For this review, take the finished solid that the model builds, in its own axes (mm). A direction names the side the tool comes from. Round coordinates to 2 decimals unless told otherwise and drop trailing zeros. Loops run counter-clockwise (first coordinate to the right, second up) from the corner with the lowest first, then second, coordinate; pieces in that order, holes last. Notation, with made-up numbers: (20, -39) -> (38, -39) arc R17 cw to (38, -29) -> close; hole circle Ø3 at (48, -9). An arc over 180 degrees is marked (long way). One line per question, with ' | ' between items. Start each with the question number.
1. Consider section C-C (x = -10.5). Write out the cut boundary in (y, z).
2. For pin 1 Ø8 at (x, y) = (11.5, 5) entering from -Z, flat-tipped, find the tip position at first contact; note if it passes through.
3. Wall thickness on line 1 along Y through (x, z) = (-2, 90.5); line 2 along X through (y, z) = (11.75, 30): over which ranges is each line inside the solid? List them lowest first.
4. For faces 1 (the face through (11.1, 11.14, 105.49)), 2 (the face through (-13.196, -13.289, 105.49)), list the 3-axis set-ups (+Z, -Z, +X, -X, +Y, -Y) from which the entire face can be reached by the end or side of a thin tool; tool diameter is ignored.
5. Consider section B-B (z = 157). Write out the cut boundary in (x, y), and give its area (3 significant figures).
6. Consider section A-A (y = 6.25). Write out the cut boundary in (x, z).
7. Draft analysis for pull direction X (two halves, no side actions). For faces 3 (the face through (0, 15, 101)), 4 (the face through (13.196, 13.289, 105.489)), 5 (the face through (0, 12, 101)), state which applies: pulls with the +X half, pulls with the -X half, needs draft (parallel to the pull), parting line crosses it, or undercut.
Autodesk Inventor part; units mm, degrees
ref_plane "Start Plane" through (0, 0, 20.1246) normal (0, 0, 1) x (1, 0, 0)
ref_plane "End Plane" through (0, 0, 185) normal (0, 0, 1) x (1, 0, 0)
ref_plane "Work Plane4" through (-839, 9, 185) normal (0, 0, 1) x (1, 0, 0)
ref_plane "Start Plane" through (0, 0, 20.1246) normal (0, 0, 1) x (1, 0, 0)
ref_plane "End Plane" through (0, 0, 185) normal (0, 0, 1) x (1, 0, 0)
sketch "Sketch" plane through (0, 0, 0) normal (0, 0, 1) x (1, 0, 0)
  line L0 (-15, -9) -> (-15, 9)
  line L1 (-9, 15) -> (9, 15)
  line L2 (15, 9) -> (15, -9)
  line L3 (9, -15) -> (-9, -15)
  arc A0 (-15, -9) -> (-9, -15) centre (-9, -9) ccw
  arc A1 (-9, 15) -> (-15, 9) centre (-9, 9) ccw
  arc A2 (15, 9) -> (9, 15) centre (9, 9) ccw
  arc A3 (9, -15) -> (15, -9) centre (9, -9) ccw
  arc A4 (-9, 12) -> (-12, 9) centre (-9, 9) ccw
  line L4 (-9, 12) -> (9, 12)
  arc A5 (12, 9) -> (9, 12) centre (9, 9) ccw
  line L5 (12, 9) -> (12, -9)
  arc A6 (9, -12) -> (12, -9) centre (9, -9) ccw
  line L6 (9, -12) -> (-9, -12)
  arc A7 (-12, -9) -> (-9, -12) centre (-9, -9) ccw
  line L7 (-12, -9) -> (-12, 9)
  line L8 (0, 22.7397) -> (0, -22.7397) construction
  line L9 (-22.7397, 0) -> (22.7397, 0) construction
  dimension "d7" = 6
  dimension "d10" = 30
  dimension "d11" = 30
  dimension "d12" = 3
  dimension "d15" = 15
  dimension "d16" = 15
extrude "Body" add sketch "Sketch" along normal up to surface (164.8754 mm away) from surface at 20.1246
sketch "Sketch3" plane through (0, 0, 0) normal (0, 0, 1) x (1, 0, 0)
  line L0 (0, 0) -> (10, 0)
ref_plane "Work Plane3" through (0, 0, 0) normal (0, -1, 0) x (1, 0, 0)
ref_plane "Work Plane4" through (-839, 9, 185) normal (0, 0, 1) x (1, 0, 0)
split "Split1" plane through (-839, 9, 185) removes the side toward (0, 0, 1)
ref_plane "Work Plane5" through (-10, -9, 11.1803) normal (0.6667, 0, -0.7454) x (-0.7454, 0, -0.6667)
split "Split2" plane through (-10, -9, 11.1803) removes the side toward (0.6667, 0, -0.7454)
ref_plane "Work Plane6" through (-213.6068, -9, 211.1803) normal (-0.6667, 0, -0.7454) x (-0.7454, 0, 0.6667)
split "Split3" plane through (-213.6068, -9, 211.1803) removes the side toward (-0.6667, 0, -0.7454)
sketch "Sketch4" plane through (0, 0, 0) normal (0, -1, 0) x (1, 0, 0)
  line L0 (-2, 20.1246) -> (12, 20.1246)
  line L1 (-2, 185) -> (12, 185)
  dimension "d18" = 164.8754
equation "\"d7\" = G_IR"
equation "\"d10\" = G_H"
equation "\"d11\" = G_W"
equation "\"d12\" = G_T"
equation "\"d15\" = 0.5 * d10"
equation "\"d16\" = 0.5 * d11"
equation "\"d3\" = G_L"
equation "\"G_W\" = 30"
equation "\"G_H\" = 30"
equation "\"G_T\" = 3"
equation "\"G_IR\" = 6"
equation "\"G_L\" = d18"
equation "\"G_OFFSET_START\" = -20.12461"
equation "\"G_OFFSET_END\" = -15"
equation "\"d13\" = -G_OFFSET_START"
equation "\"d14\" = G_OFFSET_END + B_L"
properties part number "DIN EN 10219-2 - 30 x 30 x 3  - 164.88" material "Steel, Mild"
Answer block:
1) outline: (-14.81, 29.52) -> (-11.6, 29.52) -> (-11.6, 185) -> (-14.81, 185) -> close; (11.6, 29.52) -> (14.81, 29.52) -> (14.81, 185) -> (11.6, 185) -> close
2) pin 1: stops at z = 30.86
3) line 1: y = -15 to -12, 12 to 15 | line 2: x = -11.04 to -10.2, 10.2 to 11.04
4) face 1: +Z, -Z | face 2: +Z, -Z, -X, -Y
5) outline: (-15, -9) arc R6 ccw to (-9, -15) -> (9, -15) arc R6 ccw to (15, -9) -> (15, 9) arc R6 ccw to (9, 15) -> (-9, 15) arc R6 ccw to (-15, 9) -> close; hole (-12, -9) arc R3 ccw to (-9, -12) -> (9, -12) arc R3 ccw to (12, -9) -> (12, 9) arc R3 ccw to (9, 12) -> (-9, 12) arc R3 ccw to (-12, 9) -> close | area: 301 mm2
6) outline: (-15, 33.54) -> (-12, 30.86) -> (-12, 185) -> (-15, 185) -> close; (12, 30.86) -> (15, 33.54) -> (15, 185) -> (12, 185) -> close
7) face 3: needs draft | face 4: pulls with the +X half | face 5: undercut
